from build123d import *

# Parameters (mm, degrees)
SKETCH2_R           = 1.75
CUT_EXTRUDE1_DEPTH  = 17
SKETCH3_W           = 1
SKETCH3_H           = 2.5
BOSS_EXTRUDE1_DEPTH = 2
CHAMFER1_SIZE       = 0.25
BOSS_EXTRUDE2_START = -3.1
SKETCH5_R           = 4.10031535
SKETCH5_R_2         = 3.83
BOSS_EXTRUDE2_DEPTH = 3.1


with BuildPart() as part:
    # Sketch1 → Revolve1 (revolve)
    with BuildSketch(Plane(origin=(0, 0, 0), x_dir=(1, 0, 0), z_dir=(0, 1, 0))):
        Polygon((0, 0), (0, 3), (2.5, 3), (2.5, 3.83), (19, 3.83), (19, 0), align=None)
    revolve(axis=Axis((19, 0, 0), (-1, 0, 0)))

    # Sketch2 → Cut-Extrude1 (cut)
    with BuildSketch(Plane.ZY):
        Circle(SKETCH2_R)
    extrude(amount=-CUT_EXTRUDE1_DEPTH, mode=Mode.SUBTRACT)

    # Sketch3 → Boss-Extrude1 (add)
    with BuildSketch(Plane(origin=(19, 0, 0), x_dir=(0, 0, -1), z_dir=(1, 0, 0))):
        with Locations((-1.5, 0)):
            Rectangle(SKETCH3_W, SKETCH3_H)
        with Locations((1.5, 0)):
            Rectangle(SKETCH3_W, SKETCH3_H)
    extrude(amount=BOSS_EXTRUDE1_DEPTH)

    # Chamfer1
    chamfer1_edges = [part.edges().sort_by_distance(p)[0] for p in [
        (0, 0, -1.75),
        (19, 0, 3.83),
        (0, 0, 3),
    ]]
    chamfer(chamfer1_edges, length=CHAMFER1_SIZE)

    # Sketch5 → Boss-Extrude2 (add)
    with BuildSketch(Plane.ZY.offset(-2.5).offset(BOSS_EXTRUDE2_START)):
        Circle(SKETCH5_R)
        with Locations(Location((0, 0, 0), (0, 0, 180))):
            Circle(SKETCH5_R_2, mode=Mode.SUBTRACT)
    extrude(amount=BOSS_EXTRUDE2_DEPTH)


solid = part.part
Could you check a few things on this model? Use its own coordinates, in mm. A direction names the side the tool comes from. Coordinates: 2 decimals unless noted, no trailing zeros. Loops run counter-clockwise (first coordinate to the right, second up) from the corner with the lowest first, then second, coordinate; pieces in that order, holes last.
1. Imagine slicing it at A-A (z = 0). Please give me the cut outline in (x, y).
2. Imagine slicing it at D-D (x = 1.75). Please give me the cut outline in (y, z).
3. We'd pull the mould along Y, two halves only. Please class faces 1 (the face through (17, 0, 0)), 2 (the face through (20, 0, 2)), 3 (the face through (4.07, 1.23, 3.91)): released by +Y, released by -Y, zero draft, split by the parting line, or undercut.
4. Imagine slicing it at C-C (x = 13.25). Please give me the cut outline in (y, z).
5. For faces 4 (the face through (20, 0, 1)), 5 (the face through (20, 1.25, -1.5)), 6 (the face through (2.5, -1, -3)), 7 (the face through (20, 0, -2)), which set-ups out of +Z, -Z, +X, -X, +Y, -Y let a thin tool reach every point of the face, with its end or its side?
6. I need wall thicknesses on L1, parallel to Y at x = 10.5, z = 0; L2, parallel to X at y = -3.25, z = 1.25; L3, parallel to X at y = 1.25, z = -0.5. Which ranges of each line are inside material? Lowest first, please.
7. For P1, Ø1.5, axis at y = 3, z = -3, coming from the +X side; P2, Ø0.8, axis at x = 20.5, z = -1.5, coming from the -Y side; P3, Ø1.6, axis at x = 19.5, y = -0.5, coming from the +Z side; P4, Ø2, axis at y = -2, z = 1, coming from the -X side, each with a flat end and sliding along its axis, tell me the tip position at first contact or that it passes through.
Computed values:
1. outline: (0, -2.75) - (0.25, -3) - (2.5, -3) - (2.5, -4.1) - (5.6, -4.1) - (5.6, -3.83) - (18.75, -3.83) - (19, -3.58) - (19, 3.58) - (18.75, 3.83) - (5.6, 3.83) - (5.6, 4.1) - (2.5, 4.1) - (2.5, 3) - (0.25, 3) - (0, 2.75) - (0, 2) - (0.25, 1.75) - (17, 1.75) - (17, -1.75) - (0.25, -1.75) - (0, -2) - close
2. outline: circle Ø6 at (0, 0); hole circle Ø3.5 at (0, 0)
3. face 1: undercut
3. face 2: zero draft
3. face 3: split by the parting line
4. outline: circle Ø7.66 at (0, 0); hole circle Ø3.5 at (0, 0)
5. face 4: +X, +Y, -Y
5. face 5: +Z, -Z, +X, +Y
5. face 6: -X
5. face 7: -Z, +X, +Y, -Y
6. L1: y = -3.83 to -1.75, 1.75 to 3.83
6. L2: x = 2.5 to 19
6. L3: x = 17 to 19
7. P1: stops at x = 19
7. P2: stops at y = -1.25
7. P3: stops at z = 3.82
7. P4: stops at x = 0
